Design review of the part built by this model. Coordinates are the model's own, in mm. Coordinates: 2 decimals unless noted, no trailing zeros. Order: outer loops, then holes, each group sorted by start corner. A loop starts at its lowest first (then second) coordinate and runs counter-clockwise, first axis right, second up. Notation, with made-up numbers: M 30.25,-38.5 L 45.25,-38.5 A23 cw 45.25,-5.5 Z; hole C 72,23 d7. An arc over 180 degrees is marked long. Answer as a JSON object with one key per item and string values.
Autodesk Inventor part; units mm, degrees
ref_plane "YZ Plane" through (0, 0, 0) normal (1, 0, 0) x (0, 1, 0)
ref_plane "XZ Plane" through (0, 0, 0) normal (0, 1, 0) x (-1, 0, 0)
ref_plane "XY Plane" through (0, 0, 0) normal (0, 0, 1) x (1, 0, 0)
sketch "Sketch1" plane through (0, 0, 0) normal (1, 0, 0) x (0, 1, 0)
  line L0 (0, 0) -> (25.4, 0)
  line L1 (25.4, 0) -> (25.4, -3.2512)
  line L2 (3.2512, -25.4) -> (0, -25.4)
  line L3 (0, -25.4) -> (0, 0)
  line L4 (25.4, -3.2512) -> (3.2512, -3.2512)
  line L5 (3.2512, -3.2512) -> (3.2512, -25.4)
  dimension "d2" = 3.2512
  dimension "d3" = 3.2512
  dimension "d4" = 25.4
extrude "Extrusion1" add sketch "Sketch1" along normal blind 1828.8
sketch "Sketch2" plane through (0, 0, 0) normal (0, 0, 1) x (1, 0, 0)
  line L0 (0, 0) -> (0, 25.4)
  line L1 (2.7844, 15.9512) -> (73.6304, 15.9512) construction
  circle A0 centre (12.7, 15.9512) radius 3.175
  circle A1 centre (38.1, 15.9512) radius 3.175
  line L2 (0, 25.4) -> (1828.8, 25.4)
  line L3 (0, 0) -> (1828.8, 0)
  dimension "d7" = 6.35
  dimension "d8" = 12.7
  dimension "d9" = 38.1
  dimension "d20" = 15.9512
extrude "Extrusion2" cut sketch "Sketch2" against normal blind 1828.8
sketch "Sketch3" plane through (0, 0, -25.4) normal (0, -1, 0) x (1, 0, 0)
  line L0 (1.3644, 9.4488) -> (86.9618, 9.4488) construction
  circle A0 centre (266.7, 9.4488) radius 3.175
  circle A1 centre (292.1, 9.4488) radius 3.175
  line L1 (0, 25.4) -> (1828.8, 25.4)
  line L2 (0, 0) -> (0, 25.4)
  circle A2 centre (215.9, 9.4488) radius 3.175
  dimension "d12" = 6.35
  dimension "d17" = 15.9512
  dimension "d18" = 266.7
  dimension "d19" = 292.1
  dimension "d31" = 215.9
extrude "Extrusion3" cut sketch "Sketch3" against normal blind 1828.8
sketch "Sketch4" plane through (0, 0, 0) normal (0, 0, 1) x (1, 0, 0)
  line L0 (1828.8, 25.4) -> (1828.8, 0)
  line L1 (1828.8, 12.7) -> (1190.8061, 12.7) construction
  circle A0 centre (1816.1, 12.7) radius 3.175
  circle A1 centre (1689.1, 12.7) radius 3.175
  point P0 (0, 0)
  dimension "d21" = 6.35
  dimension "d22" = 12.7
  dimension "d23" = 139.7
extrude "Extrusion4" cut sketch "Sketch4" against normal blind 1828.8
sketch "Sketch5" plane through (0, 0, -25.4) normal (0, -1, 0) x (1, 0, 0)
  line L0 (1828.8, 0) -> (1828.8, 22.1488)
  line L1 (1828.8, 11.0744) -> (1744.1467, 11.0744) construction
  circle A0 centre (1689.1, 11.0744) radius 3.175
  circle A1 centre (1816.1, 11.0744) radius 3.175
  point P0 (0, 25.4)
  dimension "d26" = 6.35
  dimension "d27" = 12.7
  dimension "d28" = 139.7
extrude "Extrusion5" cut sketch "Sketch5" against normal blind 1828.8
properties part number "Lower Long L"
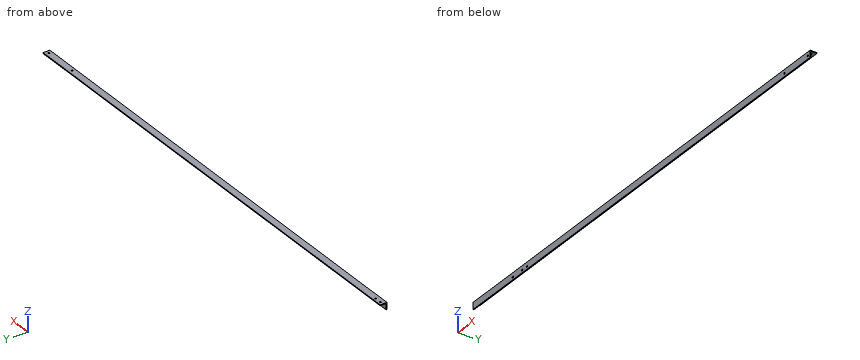
1) To check wall thickness, follow L1, parallel to Y at x = 38.1, z = -0.95; L2, parallel to Z at x = 292.1, y = 2.4; L3, parallel to Y at x = 1689.1, z = -1.4 (3 decimals). State the ranges of each line that lie inside material, in increasing order.
Taken from the geometry:
{"L1": "y = 0 to 12.78, 19.13 to 25.4", "L2": "z = -25.4 to -19.13, -12.78 to 0", "L3": "y = 0 to 9.525, 15.875 to 25.4"}
2) Insertion check: pin 1 Ø2 at (x, z) = (443, -18.5) entering from -Y; pin 2 Ø5 at (x, y) = (1308, 18) entering from -Z; pin 3 Ø6.5 at (x, z) = (656, -14.5) entering from +Y. Each pin has a flat end and moves straight along its axis. Give the tip position at first contact, or say it passes through.
Taken from the geometry:
{"pin 1": "stops at y = 0", "pin 2": "stops at z = -3.25", "pin 3": "stops at y = 3.25"}
3) Add section A-A (x = 1223.5). State the section outline as (y, z) points, and give its area (3 significant figures).
Taken from the geometry:
{"outline": "M 0,-25.4 L 3.25,-25.4 L 3.25,-3.25 L 25.4,-3.25 L 25.4,0 L 0,0 Z", "area": "155 mm2"}
